Check sheet for the modelled part. Datum: model origin and axes. Units: mm. A direction names the side the tool comes from. Round coordinates to 2 decimals unless told otherwise and drop trailing zeros. Order: outer loops, then holes, each group sorted by start corner. A loop starts at its lowest first (then second) coordinate and runs counter-clockwise, first axis right, second up. Notation, with made-up numbers: (63.25, 53.25) -> (120.25, 53.25) arc R31 ccw to (120.25, 81.25) -> close; hole circle Ø9 at (-4.5, 18). An arc over 180 degrees is marked (long way). Answer in a Markdown table with one row per item. Add a question column.
1. Draft check along Y on faces 1 (the flat face through (13.054, -38, -32)), 2 (the flat face through (-3, -50.8, -24)), 3 (the flat face through (-3, 0, -2)), 4 (the flat face through (-68.27, -30.69, -19.93)). Enter one of: +Y half, -Y half, draft (parallel to the pull), parting line (faces both ways), or undercut.
2. Access from +Z, -Z, +X, -X, +Y, -Y to the whole of each face (thin tool, end or side, straight path). Record for faces 5 (the flat face through (64, -25.4, 19)), 6 (the flat face through (48.346, -13, 28)), 7 (the flat face through (16, -25.4, -10)).
3. Depth check by flat-ended pin: P1, Ø3, axis at x = 7.5, y = -48.5, coming from the +Z side; P2, Ø1.6, axis at x = 13.5, z = -21, coming from the -Y side; P3, Ø5, axis at y = -44, z = -31.5, coming from the -X side. Enter the tip coordinate at first touch or a pass-through.
4. Sectioned sample at B-B, the plane x = -67.5. Record the boundary of the cut face in (y, z), then the cut area to 3 significant figures.
5. Material ranges on L1, parallel to X at y = -3, z = 26; L2, parallel to Z at x = 23, y = -18.5; L3, parallel to Y at x = -56, z = -3, recorded low to high. Write a range as from..to.
6. Sectioned sample at C-C, the plane y = -19. Record the boundary of the cut face in (x, z).
7. Sectioned sample at D-D, the plane y = -31.5. Record the boundary of the cut face in (x, z) (1 decimal).
8. Sectioned sample at A-A, the plane z = 25. Record the boundary of the cut face in (x, y), then the cut area to 3 significant figures.
```python
from build123d import *

# Parameters (mm, degrees)
F1_DEPTH = 50.8
F3_DEPTH = 25.4
F4_W     = 58.468216
F4_H     = 5.453941
F5_DEPTH = 6.096
F6_R     = 4.379023
F6_R_2   = 1.790502
F6_R_3   = 1.715079
F6_R_4   = 3.973674
F6_W     = 7.999114
F6_H     = 1.817981
F6_W_2   = 9.089913
F7_DEPTH = 23.114
F8_R     = 3.529881
F8_R_2   = 3.317504
F8_W     = 22.542965
F8_H     = 4.544951
F9_DEPTH = 25.4


with BuildPart() as f1:
    # F0 (on Front) → F1 (new body)
    with BuildSketch(Plane.XZ):
        Polygon((48.492239, 0), (-53.107761, 0), (-83.862998, -40.432109), (79.247475, -40.432109), align=None)
    extrude(amount=F1_DEPTH)

    # F2 (on Front) → F3 (join)
    with BuildSketch(Plane.XZ):
        Polygon((-83.75679, -40.292807), (-53.249381, 0), (-53.249381, 55.834316), (-83.75679, 55.834316), align=None)
        Polygon((48.34605, 55.834316), (48.34605, 0), (79.429068, -40.292807), (79.429068, 55.834316), align=None)
    extrude(amount=F3_DEPTH)

    # F4 (on face) → F5 (cut)
    with BuildSketch(Plane.XZ.offset(50.8)):
        with Locations((0, -20.114008)):
            Rectangle(F4_W, F4_H)
    extrude(amount=-F5_DEPTH, mode=Mode.SUBTRACT)

    # F6 (on face) → F7 (join)
    with BuildSketch(Plane.XZ.offset(50.8)):
        with Locations((0, -32.47628)):
            Circle(F6_R)
        with Locations((10.145307, -32.112684)):
            Circle(F6_R_2)
        with Locations((-9.670687, -32.294482)):
            Circle(F6_R_3)
        with Locations((0, -10.660506)):
            Circle(F6_R_4)
        with Locations((-18.396996, -11.569497)):
            Rectangle(F6_W, F6_H)
        with Locations((16.690036, -11.569497)):
            Rectangle(F6_W_2, F6_H)
    extrude(amount=-F7_DEPTH)

    # F8 (on face) → F9 (cut)
    with BuildSketch(Plane.XZ.offset(50.8)):
        Polygon((-3.287774, -15.02366), (3.580596, -15.02366), (5.703039, -8.491452), (0.146411, -4.454326), (-5.410217, -8.491452), align=None)
        with Locations((-17.851602, -10.29691)):
            Circle(F8_R)
        with Locations((15.962845, -10.29691)):
            Circle(F8_R_2)
        with Locations((1.782593, -31.476389)):
            Rectangle(F8_W, F8_H)
    extrude(amount=-F9_DEPTH, mode=Mode.SUBTRACT)


solid = f1.part
```
Answer key:
| question | item | result |
|---|---|---|
| 1 | face 1 | draft |
| 1 | face 2 | -Y half |
| 1 | face 3 | +Y half |
| 1 | face 4 | undercut |
| 2 | face 5 | +Z, +X, -Y |
| 2 | face 6 | +Z, +Y, -Y |
| 2 | face 7 | -Y |
| 3 | P1 | stops at z = 0 |
| 3 | P2 | stops at y = -44.7 |
| 3 | P3 | stops at x = -78.97 |
| 4 | outline | (-50.8, -40.43) -> (0, -40.43) -> (0, -18.92) -> (-50.8, -18.92) -> close; (-25.4, -18.82) -> (0, -18.82) -> (0, 55.83) -> (-25.4, 55.83) -> close |
| 4 | area | 2,990 mm² |
| 5 | L1 | x = -83.76..-53.25, 48.35..79.43 |
| 5 | L2 | z = -40.43..0 |
| 5 | L3 | y = -25.4..0 |
| 6 | outline | (-83.86, -40.43) -> (79.25, -40.43) -> (58.82, -13.58) -> (79.43, -40.29) -> (79.43, 55.83) -> (48.35, 55.83) -> (48.35, 0) -> (-53.11, 0) -> (-83.7, -40.22) -> (-53.25, 0) -> (-53.25, 55.83) -> (-83.76, 55.83) -> (-83.76, -40.29) -> close |
| 7 | outline | (-83.9, -40.4) -> (79.2, -40.4) -> (48.5, 0) -> (-53.1, 0) -> close; hole circle Ø7.1 at (-17.9, -10.3); hole (-9.5, -33.7) -> (13.1, -33.7) -> (13.1, -29.2) -> (-9.5, -29.2) -> close; hole (-5.4, -8.5) -> (-3.3, -15) -> (3.6, -15) -> (5.7, -8.5) -> (0.1, -4.5) -> close; hole circle Ø6.6 at (16, -10.3) |
| 8 | outline | (-83.76, -25.4) -> (-53.25, -25.4) -> (-53.25, 0) -> (-83.76, 0) -> close; (48.35, -25.4) -> (79.43, -25.4) -> (79.43, 0) -> (48.35, 0) -> close |
| 8 | area | 1,560 mm² |
